CAD build for the part. Positions are in the model's coordinates, mm. A direction names the side the tool comes from. Round coordinates to 2 decimals unless told otherwise and drop trailing zeros. Loops run counter-clockwise (first coordinate to the right, second up) from the corner with the lowest first, then second, coordinate; pieces in that order, holes last. Notation, with made-up numbers: M 5.5,59 L 29.5,59 A28 ccw 29.5,81 Z; hole C -37,89 d3. An arc over 180 degrees is marked long. Put each result on its own line as item: value. Start each with the question number.
from build123d import *

# Parameters (mm, degrees)
F0_R     = 6.5
F0_R_2   = 2
F0_R_3   = 2.1
F1_DEPTH = 1.5
F2_R     = 15
F3_R     = 20
F4_R     = 5


with BuildPart() as f1:
    # F0 (on Right) → F1 (new body, symmetric)
    with BuildSketch(Plane.YZ):
        with BuildLine():
            ThreePointArc((15.9438017453, 21.8347446946), (10.092966313, 26.4624215835), (4.5911055058, 31.5))
            ThreePointArc((4.5911055058, 31.5), (-6.9088944942, 20), (4.5911055058, 8.5))
            ThreePointArc((4.5911055058, 8.5), (12.7228334895, 11.8682720164), (16.0911055058, 20))
            ThreePointArc((16.0911055058, 20), (16.0542204131, 20.9203241946), (15.9438017453, 21.8347446946))
        make_face()
        with Locations((4.5911055058, 20)):
            Circle(F0_R, mode=Mode.SUBTRACT)
        with BuildLine():
            ThreePointArc((15.9438017453, 21.8347446946), (12.0459843114, 28.7564137633), (4.5911055058, 31.5))
            ThreePointArc((4.5911055058, 31.5), (10.092966313, 26.4624215835), (15.9438017453, 21.8347446946))
        make_face()
        with BuildLine():
            ThreePointArc((16.0911055058, 20), (12.7228334895, 11.8682720164), (4.5911055058, 8.5))
            ThreePointArc((4.5911055058, 8.5), (9.6606547276, 0), (4.5911055058, -8.5))
            ThreePointArc((4.5911055058, -8.5), (12.7228334895, -11.8682720164), (16.0911055058, -20))
            ThreePointArc((16.0911055058, -20), (16.0542204131, -20.9203241946), (15.9438017453, -21.8347446946))
            ThreePointArc((15.9438017453, -21.8347446946), (32.9549775317, -11.7027354234), (51.585894078, -5))
            Line((51.585894078, -5), (80.585894078, -5))
            Line((80.585894078, -5), (80.585894078, 5))
            Line((80.585894078, 5), (51.585894078, 5))
            ThreePointArc((51.585894078, 5), (32.9549775317, 11.7027354234), (15.9438017453, 21.8347446946))
            ThreePointArc((15.9438017453, 21.8347446946), (16.0542204131, 20.9203241946), (16.0911055058, 20))
        make_face()
        with Locations((20.9452081472, -7)):
            Circle(F0_R_2, mode=Mode.SUBTRACT)
        with Locations((20.9452081472, 7)):
            Circle(F0_R_2, mode=Mode.SUBTRACT)
        with Locations((39.085894078, 0)):
            Circle(F0_R_2, mode=Mode.SUBTRACT)
        with Locations((58.825894078, 0)):
            Circle(F0_R_3, mode=Mode.SUBTRACT)
        with Locations((69.825894078, 0)):
            Circle(F0_R_3, mode=Mode.SUBTRACT)
        with BuildLine():
            ThreePointArc((16.0911055058, -20), (12.7228334895, -11.8682720164), (4.5911055058, -8.5))
            ThreePointArc((4.5911055058, -8.5), (-6.9088944942, -20), (4.5911055058, -31.5))
            ThreePointArc((4.5911055058, -31.5), (10.092966313, -26.4624215835), (15.9438017453, -21.8347446946))
            ThreePointArc((15.9438017453, -21.8347446946), (16.0542204131, -20.9203241946), (16.0911055058, -20))
        make_face()
        with Locations((4.5911055058, -20)):
            Circle(F0_R, mode=Mode.SUBTRACT)
        with BuildLine():
            ThreePointArc((15.9438017453, -21.8347446946), (10.092966313, -26.4624215835), (4.5911055058, -31.5))
            ThreePointArc((4.5911055058, -31.5), (12.0459843114, -28.7564137633), (15.9438017453, -21.8347446946))
        make_face()
    extrude(amount=F1_DEPTH, both=True)

    # F2
    f2_edges = [f1.edges().sort_by_distance(p)[0] for p in [
        (0, 51.585894, -5),
        (0, 51.585894, 5),
    ]]
    fillet(f2_edges, radius=F2_R)

    # F3
    f3_edges = [f1.edges().sort_by_distance(p)[0] for p in [
        (0, 15.943802, -21.834745),
        (0, 15.943802, 21.834745),
    ]]
    fillet(f3_edges, radius=F3_R)

    # F4
    f4_edges = [f1.edges().sort_by_distance(p)[0] for p in [
        (0, 4.591106, 8.5),
        (0, 4.591106, -8.5),
    ]]
    fillet(f4_edges, radius=F4_R)


solid = f1.part
(1) Mould opens along Z. For faces 1 (the cylindrical face through (0.021, 34.953, -10.785)), 2 (the cylindrical face through (0.021, 35.344, 10.611)), 3 (the flat face through (0, 80.586, 0)), 4 (the cylindrical face through (-0.021, 3.745, 26.445)) say: +Z half, -Z half, draft (parallel to the pull), parting line (faces both ways), or undercut.
(2) Cut at D-D on y = 65. List the corners of the cut face in (x, z), and give its area (3 significant figures).
(3) Tool access for faces 5 (the flat face through (0, 67, 5)), 6 (the flat face through (0, 67, -5)), 7 (the cylindrical face through (0.02, 9.66, 0.12)): list every direction of +Z, -Z, +X, -X, +Y, -Y with a clear straight run to the whole face (end or side of a thin tool).
(4) Cut at B-B on y = -0.5. List the corners of the cut face in (x, z), and give its area (3 significant figures).
(5) Cut at A-A on z = 0. List the corners of the cut face in (x, y), and give its area (3 significant figures).
(6) Cut at C-C on x = 0.6. Count the separate pieces of the cut face and the enclosed holes in it, and give its area (3 significant figures).
(7) Flat gauge pin, fed straight in: pin 1 Ø0.9 at (x, y) = (0, 60.5) entering from +Z. Where does the tip first touch, or does it go through?
(8) Drill centre lines: line 1 along Z through (x, y) = (-0.6, 70); line 2 along Z through (x, y) = (-0.55, 1); line 3 along Z through (x, y) = (-0.3, 7). Where is each one in solid material? Low to high.
Taken from the geometry:
1. face 1: -Z half
1. face 2: +Z half
1. face 3: draft
1. face 4: undercut
2. outline: M -1.5,-5 L 1.5,-5 L 1.5,5 L -1.5,5 Z
2. area: 30.0 mm2
3. face 5: +Z, +X, -X, +Y
3. face 6: -Z, +X, -X, +Y
3. face 7: +X, -X, -Y
4. outline: M -1.5,-30.31 L 1.5,-30.31 L 1.5,-24.04 L -1.5,-24.04 Z; M -1.5,-15.96 L 1.5,-15.96 L 1.5,-9.69 L -1.5,-9.69 Z; M -1.5,9.69 L 1.5,9.69 L 1.5,15.96 L -1.5,15.96 Z; M -1.5,24.04 L 1.5,24.04 L 1.5,30.31 L -1.5,30.31 Z
4. area: 75.2 mm2
5. outline: M -1.5,9.66 L 1.5,9.66 L 1.5,37.09 L -1.5,37.09 Z; M -1.5,41.09 L 1.5,41.09 L 1.5,56.73 L -1.5,56.73 Z; M -1.5,60.93 L 1.5,60.93 L 1.5,67.73 L -1.5,67.73 Z; M -1.5,71.93 L 1.5,71.93 L 1.5,80.59 L -1.5,80.59 Z
5. area: 176 mm2
6. separate pieces: 1
6. enclosed holes: 7
6. area: 1,840 mm2
7. pin 1: z = 5
8. line 1: -5 to -2.09, 2.09 to 5
8. line 2: -30.92 to -25.42, -14.58 to -9.08, 9.08 to 14.58, 25.42 to 30.92
8. line 3: -31.24 to -26.04, -13.96 to -6.66, 6.66 to 13.96, 26.04 to 31.24
